CAD build for the part. Positions are in the model's coordinates, mm. A direction names the side the tool comes from. Round coordinates to 2 decimals unless told otherwise and drop trailing zeros. Write each loop counter-clockwise with the first axis right and the second up, starting at its lowest first coordinate (ties: lowest second). Pieces come first, ordered by that corner, then holes. Notation, with made-up numbers: (44, 78.25) - (69, 78.25) arc R21 ccw to (69, 113.25) - close; hole circle Ø8 at (88.25, -33.75). An arc over 180 degrees is marked (long way). Put each result on its own line as item: value. Start each with the question number.
Item 1: Mould opens along Y. For faces 1 (the flat face through (-9.5, 0, 50)), 2 (the flat face through (-7.9, 0, 49)), 3 (the flat face through (0.1, -8.7, 0.8)) say: released by +Y, released by -Y, zero draft, split by the parting line, or undercut.
Item 2: Pin check, flat tip, straight feed: pin 1 Ø1 at (x, y) = (3.5, -6) entering from +Z. Stop position of the tip, or through.
Item 3: Drill centre lines: line 1 (X direction, y = -4, z = 58); line 2 (Z direction, x = -4.25, y = -8.5). Where is each one in solid material? Low to high. Write a range as from..to.
Item 4: 3-axis set-ups, long thin cutter, end or side, ignore diameter. For faces 4 (the flat face through (8.3, 0.1, 100)), 5 (the flat face through (7.9, 0, 49)): which of +Z, -Z, +X, -X, +Y, -Y reach the whole face in a straight line?
Item 5: Cut at A-A (y = -5). Give the cut face in (x, z), and give its area (3 significant figures).
Item 6: Cut at C-C (z = 27.5). Give the cut face in (x, y), and give its area (3 significant figures).
Autodesk Inventor part; units mm, degrees
ref_plane "YZ Plane" through (0, 0, 0) normal (1, 0, 0) x (0, 1, 0)
ref_plane "XZ Plane" through (0, 0, 0) normal (0, 1, 0) x (-1, 0, 0)
ref_plane "XY Plane" through (0, 0, 0) normal (0, 0, 1) x (1, 0, 0)
sketch "Sketch1" plane through (0, 0, 0) normal (0, 0, 1) x (1, 0, 0)
  line L0 (-9.3, -9.5) -> (9.3, -9.5)
  line L1 (9.5, -9.3) -> (9.5, 9.3)
  line L2 (9.3, 9.5) -> (-9.3, 9.5)
  line L3 (-9.5, 9.3) -> (-9.5, -9.3)
  line L4 (-9.5, -9.5) -> (9.5, 9.5) construction
  line L5 (9.5, -9.5) -> (-9.5, 9.5) construction
  line L6 (-7.7, 7.9) -> (7.7, 7.9)
  line L7 (7.9, 7.7) -> (7.9, -7.7)
  line L8 (7.7, -7.9) -> (-7.7, -7.9)
  line L9 (-7.9, -7.7) -> (-7.9, 7.7)
  arc A0 (-7.7, 7.9) -> (-7.9, 7.7) centre (-7.7, 7.7) ccw
  arc A1 (-7.9, -7.7) -> (-7.7, -7.9) centre (-7.7, -7.7) ccw
  arc A2 (7.7, -7.9) -> (7.9, -7.7) centre (7.7, -7.7) ccw
  arc A3 (7.9, 7.7) -> (7.7, 7.9) centre (7.7, 7.7) ccw
  arc A4 (-9.3, 9.5) -> (-9.5, 9.3) centre (-9.3, 9.3) ccw
  arc A5 (-9.5, -9.3) -> (-9.3, -9.5) centre (-9.3, -9.3) ccw
  arc A6 (9.3, -9.5) -> (9.5, -9.3) centre (9.3, -9.3) ccw
  arc A7 (9.5, 9.3) -> (9.3, 9.5) centre (9.3, 9.3) ccw
  point P0 (0, 0)
  dimension "d0" = 19
  dimension "d1" = 19
  dimension "d2" = 1.6
  dimension "d3" = 0.2
  dimension "d4" = 0.2
  dimension "d5" = 0.2
  dimension "d6" = 0.2
  dimension "d7" = 0.2
  dimension "d8" = 0.2
  dimension "d9" = 0.2
  dimension "d10" = 0.2
extrude "Extrusion1" add sketch "Sketch1" along normal blind 100
sketch "Sketch2" plane through (9.5, -9.3, 0) normal (1, 0, 0) x (0, 0, -1)
  line L0 (0, 17.2) -> (-1.6, 18.8)
  line L1 (0, 18.8) -> (-100, 18.8)
  line L2 (0, 17.2) -> (2.2627, 17.2) construction
  line L3 (-1.6, 18.8) -> (0, 18.8)
  line L4 (0, 18.8) -> (0, 17.2)
  line L5 (0, 1.4) -> (-100, 1.4)
  line L6 (0, 1.4) -> (-1.6, -0.2)
  line L7 (0, -0.2) -> (-100, -0.2)
  line L8 (0, 1.4) -> (2.2627, 1.4) construction
  line L9 (-1.6, -0.2) -> (0, -0.2)
  line L10 (0, -0.2) -> (0, 1.4)
  line L11 (0, 0) -> (0, 18.6)
  point P0 (0, 9.3)
  dimension "d13" = 135
  dimension "d14" = 135
extrude "Extrusion2" cut sketch "Sketch2" against normal through all
sketch "Sketch3" plane through (-9.3, 9.5, 100) normal (0, 1, 0) x (1, 0, 0)
  line L0 (1.3863, 100) -> (16.0747, 100) construction
  line L1 (-0.2, 98.6) -> (-0.2, 0)
  line L2 (18.8, 98.6) -> (18.8, 0)
  line L3 (1.4, 100) -> (-0.2, 98.4)
  line L4 (1.4, 100) -> (3.6627, 100) construction
  line L5 (-0.2, 98.4) -> (-0.2, 100)
  line L6 (-0.2, 100) -> (1.4, 100)
  line L7 (17.2, 100) -> (18.8, 98.4)
  line L8 (17.2, 100) -> (19.4627, 100) construction
  line L9 (18.8, 98.4) -> (18.8, 100)
  line L10 (18.8, 100) -> (17.2, 100)
  point P0 (9.3, 100)
  dimension "d18" = 135
  dimension "d19" = 45
extrude "Extrusion3" cut sketch "Sketch3" against normal through all
properties part number "WeldingDemo"
Output values:
1. face 1: zero draft
1. face 2: undercut
1. face 3: released by -Y
2. pin 1: through
3. line 1: -9.5..-7.9, 7.9..9.5
3. line 2: 0.6..100
4. face 4: +Z, +X, -X, +Y, -Y
4. face 5: +Z, -Z
5. outline: (-9.5, 1.6) - (-7.9, 0) - (-7.9, 100) - (-9.5, 100) - close; (7.9, 0) - (9.5, 1.6) - (9.5, 100) - (7.9, 100) - close
5. area: 317 mm2
6. outline: (-9.5, -9.3) arc R0.2 ccw to (-9.3, -9.5) - (9.3, -9.5) arc R0.2 ccw to (9.5, -9.3) - (9.5, 9.3) arc R0.2 ccw to (9.3, 9.5) - (-9.3, 9.5) arc R0.2 ccw to (-9.5, 9.3) - close; hole (-7.9, -7.7) arc R0.2 ccw to (-7.7, -7.9) - (7.7, -7.9) arc R0.2 ccw to (7.9, -7.7) - (7.9, 7.7) arc R0.2 ccw to (7.7, 7.9) - (-7.7, 7.9) arc R0.2 ccw to (-7.9, 7.7) - close
6. area: 111 mm2
